```python
from build123d import *

# Parameters (mm, degrees)
BOSS_EXTRUDE1_DEPTH = 5.2
FILLET1_R           = 10
BOSS_EXTRUDE2_DEPTH = 1
SKETCH2_R           = 2.5
CUT_EXTRUDE1_DEPTH  = 5.2
BOSS_EXTRUDE3_DEPTH = 20
SKETCH7_W           = 15.78
SKETCH7_H           = 10
BOSS_EXTRUDE5_DEPTH = 0.75
CUT_EXTRUDE2_DEPTH  = 10
CUT_EXTRUDE3_DEPTH  = 1.5
FILLET6_R           = 1
CHAMFER1_SIZE       = 1
CUT_EXTRUDE4_DEPTH  = 3
SKETCH11_R          = 1.4
CUT_EXTRUDE5_DEPTH  = 3.5
CHAMFER2_SIZE       = 1.4
CUT_EXTRUDE6_DEPTH  = 0.5
CHAMFER3_SIZE       = 1
SKETCH13_W          = 25.4
SKETCH13_H          = 10.2
CUT_EXTRUDE7_DEPTH  = 217.847965174
FILLET7_R           = 5.1
FILLET8_R           = 3
FILLET9_R           = 15


with BuildPart() as part:
    # Sketch1 → Boss-Extrude1 (new body)
    with BuildSketch(Plane(origin=(0, 0, 0), x_dir=(1, 0, 0), z_dir=(0, 1, 0))):
        with BuildLine():
            ThreePointArc((-106, -34), (-104.828427125, -36.828427125), (-102, -38))
            Line((-102, -38), (102, -38))
            ThreePointArc((102, -38), (104.828427125, -36.828427125), (106, -34))
            Line((106, -34), (106, 34))
            ThreePointArc((106, 34), (104.828427125, 36.828427125), (102, 38))
            Line((102, 38), (-102, 38))
            ThreePointArc((-102, 38), (-104.828427125, 36.828427125), (-106, 34))
            Line((-106, 34), (-106, -34))
        make_face()
        with BuildLine():
            ThreePointArc((-87, -33), (-91.100505063, -23.100505063), (-101, -19))
            Line((-101, -19), (-101, 19))
            ThreePointArc((-101, 19), (-91.100505063, 23.100505063), (-87, 33))
            Line((-87, 33), (87, 33))
            ThreePointArc((87, 33), (91.100505063, 23.100505063), (101, 19))
            Line((101, 19), (101, -19))
            ThreePointArc((101, -19), (91.100505063, -23.100505063), (87, -33))
            Line((87, -33), (-87, -33))
        make_face(mode=Mode.SUBTRACT)
    extrude(amount=BOSS_EXTRUDE1_DEPTH)

    # Fillet1
    fillet1_edges = [part.edges().sort_by_distance(p)[0] for p in [
        (101, 2.6, -19),
        (87, 2.6, -33),
        (-87, 2.6, -33),
        (-101, 2.6, -19),
        (-101, 2.6, 19),
        (-87, 2.6, 33),
        (87, 2.6, 33),
        (101, 2.6, 19),
    ]]
    fillet(fillet1_edges, radius=FILLET1_R)

    # Sketch3 → Boss-Extrude2 (add)
    with BuildSketch(Plane(origin=(0, 0, 0), x_dir=(-1, 0, 0), z_dir=(0, -1, 0))):
        with BuildLine():
            Line((-102, -38), (-76, -38))
            Line((-76, -38), (-76, 38))
            Line((-76, 38), (-102, 38))
            ThreePointArc((-102, 38), (-104.828427125, 36.828427125), (-106, 34))
            Line((-106, 34), (-106, -34))
            ThreePointArc((-106, -34), (-104.828427125, -36.828427125), (-102, -38))
        make_face()
        with BuildLine():
            Line((102, -38), (76, -38))
            Line((76, -38), (76, 38))
            Line((76, 38), (102, 38))
            ThreePointArc((102, 38), (104.828427125, 36.828427125), (106, 34))
            Line((106, 34), (106, -34))
            ThreePointArc((106, -34), (104.828427125, -36.828427125), (102, -38))
        make_face()
    extrude(amount=-BOSS_EXTRUDE2_DEPTH)

    # Sketch2 → Cut-Extrude1 (cut)
    with BuildSketch(Plane(origin=(0, 5.2, 0), x_dir=(1, 0, 0), z_dir=(0, 1, 0))):
        with Locations(Location((-96, 25.5, 0), (0, 0, 270))):
            Circle(SKETCH2_R)
        with Locations(Location((96, 25.5, 0), (0, 0, 90))):
            Circle(SKETCH2_R)
        with Locations(Location((96, -25.5, 0), (0, 0, 270))):
            Circle(SKETCH2_R)
        with Locations(Location((-96, -25.5, 0), (0, 0, 90))):
            Circle(SKETCH2_R)
    extrude(amount=-CUT_EXTRUDE1_DEPTH, mode=Mode.SUBTRACT)

    # Sketch4 → Boss-Extrude3 (add)
    with BuildSketch(Plane(origin=(0, 5.2, 0), x_dir=(1, 0, 0), z_dir=(0, 1, 0))):
        with BuildLine():
            Line((-102, 38), (102, 38))
            ThreePointArc((102, 38), (104.828427125, 36.828427125), (106, 34))
            Line((106, 34), (106, -34))
            ThreePointArc((106, -34), (104.828427125, -36.828427125), (102, -38))
            Line((102, -38), (-102, -38))
            ThreePointArc((-102, -38), (-104.828427125, -36.828427125), (-106, -34))
            Line((-106, -34), (-106, 34))
            ThreePointArc((-106, 34), (-104.828427125, 36.828427125), (-102, 38))
        make_face()
        with BuildLine():
            Line((102, -36), (-102, -36))
            ThreePointArc((-102, -36), (-103.414213562, -35.414213562), (-104, -34))
            Line((-104, -34), (-104, 34))
            ThreePointArc((-104, 34), (-103.414213562, 35.414213562), (-102, 36))
            Line((-102, 36), (102, 36))
            ThreePointArc((102, 36), (103.414213562, 35.414213562), (104, 34))
            Line((104, 34), (104, -34))
            ThreePointArc((104, -34), (103.414213562, -35.414213562), (102, -36))
        make_face(mode=Mode.SUBTRACT)
    extrude(amount=BOSS_EXTRUDE3_DEPTH)

    # Sketch7 → Boss-Extrude5 (add)
    with BuildSketch(Plane(origin=(0, 0, 36), x_dir=(-1, 0, 0), z_dir=(0, 0, -1))):
        with Locations((-81.5, 10.2)):
            Rectangle(SKETCH7_W, SKETCH7_H)
    extrude(amount=BOSS_EXTRUDE5_DEPTH)

    # Sketch6 → Cut-Extrude2 (cut)
    with BuildSketch(Plane.XY.offset(38)):
        with BuildLine():
            Line((84.39, 10.34), (78.61, 10.34))
            ThreePointArc((78.61, 10.34), (76.78, 8.51), (78.61, 6.68))
            Line((78.61, 6.68), (84.39, 6.68))
            ThreePointArc((84.39, 6.68), (86.22, 8.51), (84.39, 10.34))
        make_face()
    extrude(amount=-CUT_EXTRUDE2_DEPTH, mode=Mode.SUBTRACT)

    # Sketch8 → Cut-Extrude3 (cut)
    with BuildSketch(Plane.XY.offset(38)):
        with BuildLine():
            Line((78.11, 11.84), (84.89, 11.84))
            ThreePointArc((84.89, 11.84), (87.011320344, 10.961320344), (87.89, 8.84))
            Line((87.89, 8.84), (87.89, 8.18))
            ThreePointArc((87.89, 8.18), (87.011320344, 6.058679656), (84.89, 5.18))
            Line((84.89, 5.18), (78.11, 5.18))
            ThreePointArc((78.11, 5.18), (75.988679656, 6.058679656), (75.11, 8.18))
            Line((75.11, 8.18), (75.11, 8.84))
            ThreePointArc((75.11, 8.84), (75.988679656, 10.961320344), (78.11, 11.84))
        make_face()
    extrude(amount=-CUT_EXTRUDE3_DEPTH, mode=Mode.SUBTRACT)

    # Fillet6
    fillet6_edges = [part.edges().sort_by_distance(p)[0] for p in [
        (87.011320344, 10.961320344, 38),
        (81.5, 11.84, 38),
        (75.988679656, 10.961320344, 38),
        (75.11, 8.51, 38),
        (75.988679656, 6.058679656, 38),
        (81.5, 5.18, 38),
        (87.011320344, 6.058679656, 38),
        (87.89, 8.51, 38),
    ]]
    fillet(fillet6_edges, radius=FILLET6_R)

    # Chamfer1
    # the kernel refuses this chamfer: 1 mm, written as the material it takes off along each edge
    with BuildSketch(Plane(origin=(89.39, 5.2, 35.25), x_dir=(0.027495876610582105, 0, 0.999621916911297), z_dir=(0, 1, 0))) as chamfer1_piece_1_section:
        Polygon((CHAMFER1_SIZE * 0.999621916911, -CHAMFER1_SIZE * 0.0274958766106), (-CHAMFER1_SIZE * 0.0274958766106, -CHAMFER1_SIZE * 0.999621916911), (0, 0), align=None)
    chamfer1_piece_1 = extrude(amount=12.571682988, mode=Mode.PRIVATE)
    chamfer1_piece_1 = split(chamfer1_piece_1, bisect_by=Plane(origin=(89.03804089, 11.485841494, 36), z_dir=(0, 0, -1)), keep=Keep.TOP, mode=Mode.PRIVATE)
    add(chamfer1_piece_1, mode=Mode.SUBTRACT)
    with BuildSketch(Plane(origin=(73.61, 17.771682988, 35.25), x_dir=(-0.027495876610582105, 0, 0.999621916911297), z_dir=(0, -1, 0))) as chamfer1_piece_2_section:
        Polygon((CHAMFER1_SIZE * 0.999621916911, -CHAMFER1_SIZE * 0.0274958766106), (-CHAMFER1_SIZE * 0.0274958766106, -CHAMFER1_SIZE * 0.999621916911), (0, 0), align=None)
    chamfer1_piece_2 = extrude(amount=12.571682988, mode=Mode.PRIVATE)
    chamfer1_piece_2 = split(chamfer1_piece_2, bisect_by=Plane(origin=(73.96195911, 11.485841494, 36), z_dir=(0, 0, -1)), keep=Keep.TOP, mode=Mode.PRIVATE)
    add(chamfer1_piece_2, mode=Mode.SUBTRACT)

    # Sketch9 → Cut-Extrude4 (cut)
    with BuildSketch(Plane.XY.offset(38)):
        with BuildLine():
            Line((-84, 15.81), (-79, 15.81))
            ThreePointArc((-79, 15.81), (-74, 10.81), (-79, 5.81))
            Line((-79, 5.81), (-84, 5.81))
            ThreePointArc((-84, 5.81), (-89, 10.81), (-84, 15.81))
        make_face()
    extrude(amount=-CUT_EXTRUDE4_DEPTH, mode=Mode.SUBTRACT)

    # Sketch11 → Cut-Extrude5 (cut)
    with BuildSketch(Plane.XY.offset(38)):
        with Locations((-94, 10.81)):
            Circle(SKETCH11_R)
        with Locations((-69, 10.81)):
            Circle(SKETCH11_R)
    extrude(amount=-CUT_EXTRUDE5_DEPTH, mode=Mode.SUBTRACT)

    # Chamfer2
    chamfer2_edges = [part.edges().sort_by_distance(p)[0] for p in [
        (-95.4, 10.81, 38),
        (-70.4, 10.81, 38),
    ]]
    chamfer(chamfer2_edges, length=CHAMFER2_SIZE)

    # Sketch12 → Cut-Extrude6 (cut)
    with BuildSketch(Plane(origin=(0, 0, 36), x_dir=(-1, 0, 0), z_dir=(0, 0, -1))):
        with BuildLine():
            Line((69, 13.81), (94, 13.81))
            ThreePointArc((94, 13.81), (97, 10.81), (94, 7.81))
            Line((94, 7.81), (69, 7.81))
            ThreePointArc((69, 7.81), (66, 10.81), (69, 13.81))
        make_face()
    extrude(amount=-CUT_EXTRUDE6_DEPTH, mode=Mode.SUBTRACT)

    # Chamfer3
    chamfer3_edges = [part.edges().sort_by_distance(p)[0] for p in [
        (0, 5.2, 33),
        (91.100505063, 5.2, 23.100505063),
        (101, 5.2, 0),
        (91.100505063, 5.2, -23.100505063),
        (0, 5.2, -33),
        (-91.100505063, 5.2, 23.100505063),
        (-101, 5.2, 0),
        (-91.100505063, 5.2, -23.100505063),
        (84.583193019, 5.2, 31.416254115),
        (99.416254115, 5.2, 16.583193019),
        (99.416254115, 5.2, -16.583193019),
        (84.583193019, 5.2, -31.416254115),
        (-84.583193019, 5.2, 31.416254115),
        (-99.416254115, 5.2, 16.583193019),
        (-84.583193019, 5.2, -31.416254115),
        (-99.416254115, 5.2, -16.583193019),
    ]]
    chamfer(chamfer3_edges, length=CHAMFER3_SIZE)

    # Sketch13 → Cut-Extrude7 (cut, through all)
    with BuildSketch(Plane(origin=(106, 0, 0), x_dir=(0, 0, -1), z_dir=(1, 0, 0))):
        with Locations((0, 20.1)):
            Rectangle(SKETCH13_W, SKETCH13_H)
    extrude(amount=-CUT_EXTRUDE7_DEPTH, mode=Mode.SUBTRACT)

    # Fillet7
    fillet7_edges = [part.edges().sort_by_distance(p)[0] for p in [
        (-105, 15, -12.7),
        (-105, 15, 12.7),
        (105, 15, -12.7),
        (105, 15, 12.7),
    ]]
    fillet(fillet7_edges, radius=FILLET7_R)

    # Fillet8
    fillet8_edges = [part.edges().sort_by_distance(p)[0] for p in [
        (-105, 25.2, -12.7),
        (-105, 25.2, 12.7),
        (105, 25.2, -12.7),
        (105, 25.2, 12.7),
    ]]
    fillet(fillet8_edges, radius=FILLET8_R)

    # Fillet9
    fillet9_edges = [part.edges().sort_by_distance(p)[0] for p in [
        (76, 0.5, 33),
        (76, 0.5, -33),
        (-76, 0.5, 33),
        (-76, 0.5, -33),
    ]]
    fillet(fillet9_edges, radius=FILLET9_R)


solid = part.part
```
Can you work these out from the model? Positions are in its coordinate system, mm. A direction names the side the tool comes from. Coordinates: 2 decimals unless noted, no trailing zeros. Loops run counter-clockwise (first coordinate to the right, second up) from the corner with the lowest first, then second, coordinate; pieces in that order, holes last. Notation, with made-up numbers: (-26, 15) -> (8, 15) arc R25 cw to (8, 39) -> close; hole circle Ø10 at (60.25, 20.5). An arc over 180 degrees is marked (long way). Put each result on its own line as item: value. Start each with the question number.
Q1. I want a section at B-B (x = -63). Write out the boundary of the cut face in (y, z), plus the area to 3 significant figures.
Q2. I'm going to push flat-ended pins straight in: P1, Ø4.5, axis at x = 96, z = 25.5, coming from the +Y side; P2, Ø1, axis at x = 105, y = 21, coming from the -Z side; P3, Ø1, axis at x = -105.5, y = 21.5, coming from the +Z side; P4, Ø5.5, axis at x = 83, y = 9.5, coming from the +Z side. Where does each tip first touch, or does it pass through?
Q3. If I drill on line 1 (X direction, y = 2.95, z = -25.5); line 2 (Z direction, x = -33, y = 6.75); line 3 (X direction, y = 12.5, z = -9.5), over which ranges is the centre line in solid material (lowest first)? Write a range as [from, to].
Q4. I want a section at A-A (x = 10.5). Write out the boundary of the cut face in (y, z), plus the area to 3 significant figures.
Q5. For faces 4 (the face through (-71.49, 0.51, -28.72)), 5 (the face through (104.986, 16.454, -11.166)), 6 (the face through (-104, 13, 0)), which set-ups out of +Z, -Z, +X, -X, +Y, -Y let a thin tool reach every point of the face, with its end or its side?
Q6. Thinking about a two-plate mould opening in Y: for faces 1 (the face through (-74, 10.9, 37)), 2 (the face through (-8.2, 5.2, 34.5)), 3 (the face through (99.373, 2.622, 16.65)), which applies, pulls with the +Y half, pulls with the -Y half, needs draft (parallel to the pull), parting line crosses it, or undercut?
Taken from the geometry:
1. outline: (0, -38) -> (25.2, -38) -> (25.2, -36) -> (5.2, -36) -> (5.2, -34) -> (4.2, -33) -> (1, -33) -> (1, -32.87) -> (0, -32.87) -> close; (0, 32.87) -> (1, 32.87) -> (1, 33) -> (4.2, 33) -> (5.2, 34) -> (5.2, 36) -> (25.2, 36) -> (25.2, 38) -> (0, 38) -> close
1. area: 131 mm2
2. P1: passes through
2. P2: stops at z = -37.12
2. P3: stops at z = 36.65
2. P4: stops at z = 37.81
3. line 1: x = [-106, -98.5], [-93.5, -89.18], [89.18, 93.5], [98.5, 106]
3. line 2: z = [-38, -36], [36, 38]
3. line 3: x = [-106, -104], [104, 106]
4. outline: (0, -38) -> (25.2, -38) -> (25.2, -36) -> (5.2, -36) -> (5.2, -34) -> (4.2, -33) -> (0, -33) -> close; (0, 33) -> (4.2, 33) -> (5.2, 34) -> (5.2, 36) -> (25.2, 36) -> (25.2, 38) -> (0, 38) -> close
4. area: 131 mm2
5. face 4: +Y, -Y
5. face 5: +X, -X, +Y
5. face 6: +Y
6. face 1: undercut
6. face 2: pulls with the +Y half
6. face 3: needs draft
